Geometry: final body of the model. Coordinates: model frame, mm. A direction names the side the tool comes from. Coordinates: 2 decimals unless noted, no trailing zeros. Loops run counter-clockwise (first coordinate to the right, second up) from the corner with the lowest first, then second, coordinate; pieces in that order, holes last. Notation, with made-up numbers: (18.25, -13) - (70.25, -13) arc R33 cw to (70.25, 25) - close; hole circle Ø5 at (-36.75, 38.5). An arc over 180 degrees is marked (long way). Return JSON: item names as keys, results as strings.
from build123d import *

# Parameters (mm, degrees)
F1_DEPTH = 20
F2_R     = 12.75
F3_DEPTH = 12
F4_R     = 10
F5_DEPTH = 2


with BuildPart() as f1:
    # F0 (on Top) → F1 (new body)
    with BuildSketch(Plane.XY):
        Polygon((0.001339, 15.588457), (-13.499331, 7.795388), (-13.500669, -7.793069), (-0.001339, -15.588457), (13.499331, -7.795388), (13.500669, 7.793069), align=None)
    extrude(amount=F1_DEPTH)

    # F2 (on Top) → F3 (cut)
    with BuildSketch(Plane.XY):
        Circle(F2_R)
    extrude(amount=F3_DEPTH, mode=Mode.SUBTRACT)

    # F4 (on face) → F5 (join)
    with BuildSketch(Plane.XY.offset(20)):
        Circle(F4_R)
    extrude(amount=F5_DEPTH)


solid = f1.part
Item 1: Mould query, pull axis X, two halves, no side actions, for faces 4 (the face through (0, 0, 12)), 5 (the face through (6.845, 11.636, 9.86)), 6 (the face through (-0.2, -10.2, 20)). Classes: +X half, -X half, draft (parallel to the pull), parting line (faces both ways), or undercut.
Worked out:
{"face 4": "undercut", "face 5": "+X half", "face 6": "draft"}
Item 2: Section query B-B, the plane y = 0. Return loops of the section in (x, z), and give its area (3 significant figures).
Worked out:
{"outline": "(-13.5, 0) - (-12.75, 0) - (-12.75, 12) - (12.75, 12) - (12.75, 0) - (13.5, 0) - (13.5, 20) - (10, 20) - (10, 22) - (-10, 22) - (-10, 20) - (-13.5, 20) - close", "area": "274 mm^2"}
Item 3: First-contact query: pin 1 Ø7.5 at (x, y) = (-1.5, -4) entering from -Z; pin 2 Ø12 at (y, z) = (9, 10) entering from -X; pin 3 Ø5 at (x, z) = (7, 13) entering from +Y; pin 4 Ø1.5 at (x, z) = (9, 2.5) entering from +Y. Flat tips, straight axial feed; report the tip coordinate or a pass-through.
Worked out:
{"pin 1": "z = 12", "pin 2": "x = -13.5", "pin 3": "y = 12.99", "pin 4": "y = 10.83"}
Item 4: Section query A-A, the plane z = 9.75. Return loops of the section in (x, y).
Worked out:
{"outline": "(-13.5, -7.79) - (0, -15.59) - (13.5, -7.8) - (13.5, 7.79) - (0, 15.59) - (-13.5, 7.8) - close; hole circle Ø25.5 at (0, 0)"}
Item 5: Ray query, probe 1 along Y at (x, z) = (0, 8); probe 2 along Z at (x, y) = (1.75, -12); probe 3 along Z at (x, y) = (-2.5, -14). Return the intervals inside material, ascending. Write a range as from..to.
Worked out:
{"probe 1": "-15.59..-12.75, 12.75..15.59", "probe 2": "12..20", "probe 3": "0..20"}
Item 6: Reachability of faces 1 (the face through (0, 0, 22)), 2 (the face through (-2.764, -12.447, 5.916)), 3 (the face through (-2.17, -9.76, 20.99)) from +Z, -Z, +X, -X, +Y, -Y: full face, straight path, thin tool, end or side. Return the list, or none.
Worked out:
{"face 1": "+Z, +X, -X, +Y, -Y", "face 2": "-Z", "face 3": "+Z"}
Item 7: Section query C-C, the plane z = 16.5. Return loops of the section in (x, y), and give its area (3 significant figures).
Worked out:
{"outline": "(-13.5, -7.79) - (0, -15.59) - (13.5, -7.8) - (13.5, 7.79) - (0, 15.59) - (-13.5, 7.8) - close", "area": "631 mm^2"}
Item 8: Section query D-D, the plane x = 9.5. Return loops of the section in (y, z), and give its area (3 significant figures).
Worked out:
{"outline": "(-10.1, 0) - (-8.5, 0) - (-8.5, 12) - (8.5, 12) - (8.5, 0) - (10.1, 0) - (10.1, 20) - (3.12, 20) - (3.12, 22) - (-3.12, 22) - (-3.12, 20) - (-10.1, 20) - close", "area": "213 mm^2"}
